```python
from build123d import *

# Parameters (mm, degrees)
SALIENTE_EXTRUIR1_DEPTH = 50
CROQUIS7_R              = 2.5
CORTAR_EXTRUIR1_DEPTH   = 5
CROQUIS8_R              = 4
SALIENTE_EXTRUIR2_DEPTH = 5
SALIENTE_EXTRUIR3_START = 5
CROQUIS15_R             = 4
SALIENTE_EXTRUIR3_DEPTH = 5
CROQUIS17_R             = 1.625
CORTAR_EXTRUIR4_DEPTH   = 6
CORTAR_EXTRUIR5_START   = -6
CROQUIS16_R             = 1.625
CORTAR_EXTRUIR5_DEPTH   = 6


with BuildPart() as part:
    # Croquis3 → Saliente-Extruir1 (new body)
    with BuildSketch(Plane(origin=(0, 0, 0), x_dir=(1, 0, 0), z_dir=(0, 1, 0))):
        Polygon((0, 0), (20.000000004, 20), (50.000000004, 20), (50.000000004, -20), (20.000000004, -20), align=None)
        Polygon((7.071067811, 2e-09), (22.071067819, 15), (45.000000004, 15), (45.000000004, -15), (22.071067815, -15), align=None, mode=Mode.SUBTRACT)
    extrude(amount=SALIENTE_EXTRUIR1_DEPTH)

    # Croquis7 → Cortar-Extruir1 (cut)
    with BuildSketch(Plane(origin=(50.000000004, 0, 0), x_dir=(0, 0, -1), z_dir=(1, 0, 0))):
        with Locations((0, 25)):
            Circle(CROQUIS7_R)
    extrude(amount=-CORTAR_EXTRUIR1_DEPTH, mode=Mode.SUBTRACT)

    # Croquis8 → Saliente-Extruir2 (add)
    with BuildSketch(Plane.XY.offset(20)):
        with Locations((35.000000004, 25)):
            Circle(CROQUIS8_R)
    extrude(amount=SALIENTE_EXTRUIR2_DEPTH)

    # Croquis15 → Saliente-Extruir3 (add)
    with BuildSketch(Plane(origin=(0, 0, -20), x_dir=(-1, 0, 0), z_dir=(0, 0, -1)).offset(SALIENTE_EXTRUIR3_START)):
        with Locations(Location((-35.000000004, 25, 0), (0, 0, 180))):
            Circle(CROQUIS15_R)
    extrude(amount=-SALIENTE_EXTRUIR3_DEPTH)

    # Croquis17 → Cortar-Extruir4 (cut)
    with BuildSketch(Plane.XY.offset(25)):
        with Locations((35.000000004, 25)):
            Circle(CROQUIS17_R)
    extrude(amount=-CORTAR_EXTRUIR4_DEPTH, mode=Mode.SUBTRACT)

    # Croquis16 → Cortar-Extruir5 (cut)
    with BuildSketch(Plane(origin=(0, 0, -25), x_dir=(-1, 0, 0), z_dir=(0, 0, -1)).offset(CORTAR_EXTRUIR5_START)):
        with Locations(Location((-35.000000004, 25, 0), (0, 0, 180))):
            Circle(CROQUIS16_R)
    extrude(amount=CORTAR_EXTRUIR5_DEPTH, mode=Mode.SUBTRACT)


solid = part.part
```
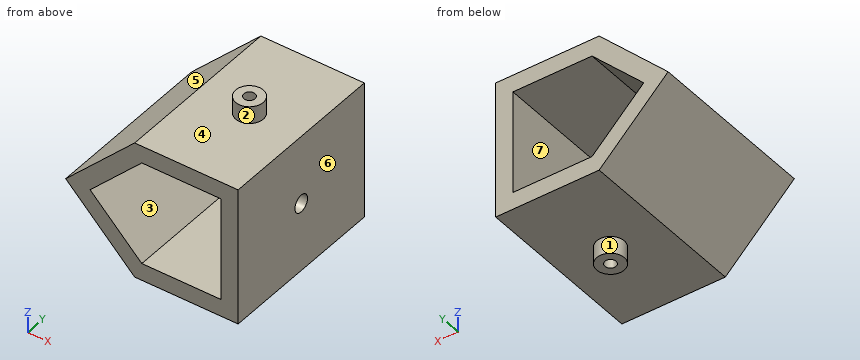
Model file for the job. Use its own axes, mm. Face numbers are marked on the shaded views. A direction names the side the tool comes from. Coordinates: 2 decimals unless noted, no trailing zeros. Write each loop counter-clockwise with the first axis right and the second up, starting at its lowest first coordinate (ties: lowest second). Pieces come first, ordered by that corner, then holes. Notation, with made-up numbers: (15.5, 20) - (63.5, 20) arc R26 cw to (63.5, 45) - close; hole circle Ø6 at (36.25, -18). An arc over 180 degrees is marked (long way). One line per question, with ' | ' between items. Start each with the question number.
Q1. 3-axis set-ups, long thin cutter, end or side, ignore diameter. For the marked faces 1, 2 and 3: which of +Z, -Z, +X, -X, +Y, -Y reach the whole face in a straight line?
Q2. Pull direction X, two halves, no side cores. Call the marked faces 4, 5, 6 and 7: pulls with the +X half, pulls with the -X half, needs draft (parallel to the pull), parting line crosses it, or undercut.
Q3. Cut at A-A, the plane x = 42.5. List the corners of the cut face in (y, z).
Q4. Drill centre lines: line 1 (Z direction, x = 42, y = 48); line 2 (Y direction, x = 47.5, z = 0); line 3 (Y direction, x = 35, z = -22.95) (3 decimals). Where is each one in solid material? Low to high. Write a range as [from, to].
Q5. Pin check, flat tips, straight feed: pin 1 (1 mm diameter, centred on x = 34.5, y = 25.5, fed in from -Z); pin 2 (25 mm diameter, centred on x = 36.5, y = 25, fed in from -Z); pin 3 (1.6 mm diameter, centred on x = 34.5, y = 25.5, fed in from +Z); pin 4 (12 mm diameter, centred on x = 25, y = 29.5, fed in from -Z). Stop position of each tip, or through.
Q6. Cut at C-C, the plane y = 7.5. List the corners of the cut face in (x, z).
Q7. Cut at B-B, the plane z = 5.5. List the corners of the cut face in (x, y).
Answer below:
1) face 1: -Z | face 2: +Z | face 3: +Y, -Y
2) face 4: needs draft | face 5: pulls with the -X half | face 6: pulls with the +X half | face 7: undercut
3) outline: (0, -20) - (50, -20) - (50, -15) - (0, -15) - close; (0, 15) - (50, 15) - (50, 20) - (0, 20) - close
4) line 1: [-20, -15], [15, 20] | line 2: [0, 22.5], [27.5, 50] | line 3: [21, 23.375], [26.625, 29]
5) pin 1: z = -19 | pin 2: z = -25 | pin 3: z = 19 | pin 4: z = -20
6) outline: (0, 0) - (20, -20) - (50, -20) - (50, 20) - (20, 20) - close; hole (7.07, 0) - (22.07, -15) - (45, -15) - (45, 15) - (22.07, 15) - close
7) outline: (5.5, 0) - (12.57, 0) - (12.57, 50) - (5.5, 50) - close; (45, 0) - (50, 0) - (50, 50) - (45, 50) - close
